The drawing under review shows one solid part. Ordinate dimensions are in mm from its lowest x, y, z. A direction names the side the tool comes from. Coordinates: 2 decimals unless noted, no trailing zeros. Loops run counter-clockwise (first coordinate to the right, second up) from the corner with the lowest first, then second, coordinate; pieces in that order, holes last. Notation, with made-up numbers: M -27,47.5 L 0,47.5 A13 cw 0,52.5 Z; hole C 3.5,75.25 d3. An arc over 180 degrees is marked long. Put each result on its own line as item: value.
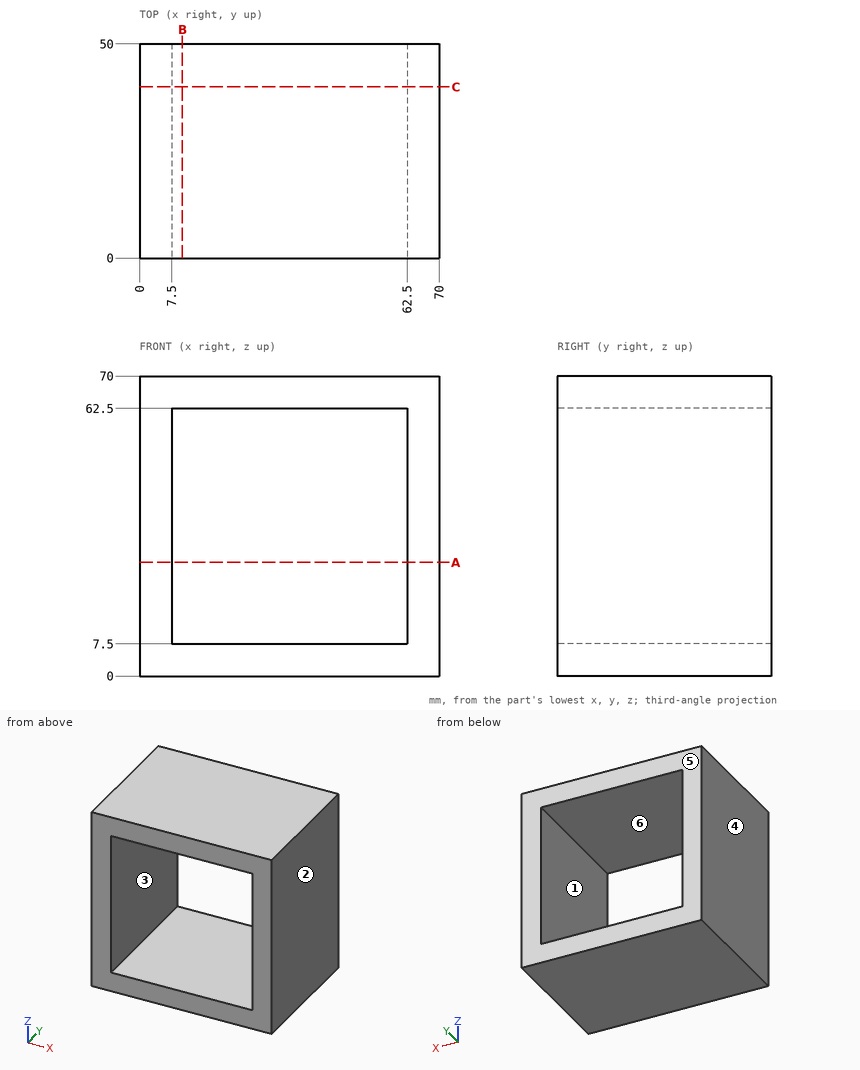
(1) Add section C-C (y = 40). Write out the cut boundary in (x, z), plus the area to 4 significant figures.
Determined:
outline: M 0,0 L 70,0 L 70,70 L 0,70 Z; hole M 7.5,7.5 L 62.5,7.5 L 62.5,62.5 L 7.5,62.5 Z
area: 1,875 mm^2
(2) Draft analysis for pull direction X (two halves, no side actions). For the marked faces 1, 2, 3 and 4, state which applies: +X half, -X half, draft (parallel to the pull), parting line (faces both ways), or undercut.
Determined:
face 1: undercut
face 2: +X half
face 3: undercut
face 4: -X half
(3) Add section B-B (x = 10). Write out the cut boundary in (y, z), plus the area to 3 significant figures.
Determined:
outline: M 0,0 L 50,0 L 50,7.5 L 0,7.5 Z; M 0,62.5 L 50,62.5 L 50,70 L 0,70 Z
area: 750 mm^2
(4) Tool access review of the marked faces 5 and 6: name each direction out of +Z, -Z, +X, -X, +Y, -Y from which nothing blocks a thin tool from reaching the whole face with its end or side.
Determined:
face 5: +Z, -Z, +X, -X, +Y
face 6: +Y, -Y
(5) For pin 1 (8 mm diameter, centred on x = 11, z = 30.5, fed in from -Y); pin 2 (4 mm diameter, centred on x = 10.5, z = 24.5, fed in from +Y), all flat-tipped, find the tip position at first contact; note any pin that passes through.
Determined:
pin 1: stops at y = 0
pin 2: passes through
(6) Wall thickness on line 1 along Z through (x, y) = (33, 7.5): over which ranges is the line inside the solid? List them lowest first. Write a range as [from, to].
Determined:
line 1: z = [0, 7.5], [62.5, 70]
(7) Add section A-A (z = 26.5). Write out the cut boundary in (x, y), plus the area to 3 significant figures.
Determined:
outline: M 0,0 L 7.5,0 L 7.5,50 L 0,50 Z; M 62.5,0 L 70,0 L 70,50 L 62.5,50 Z
area: 750 mm^2
